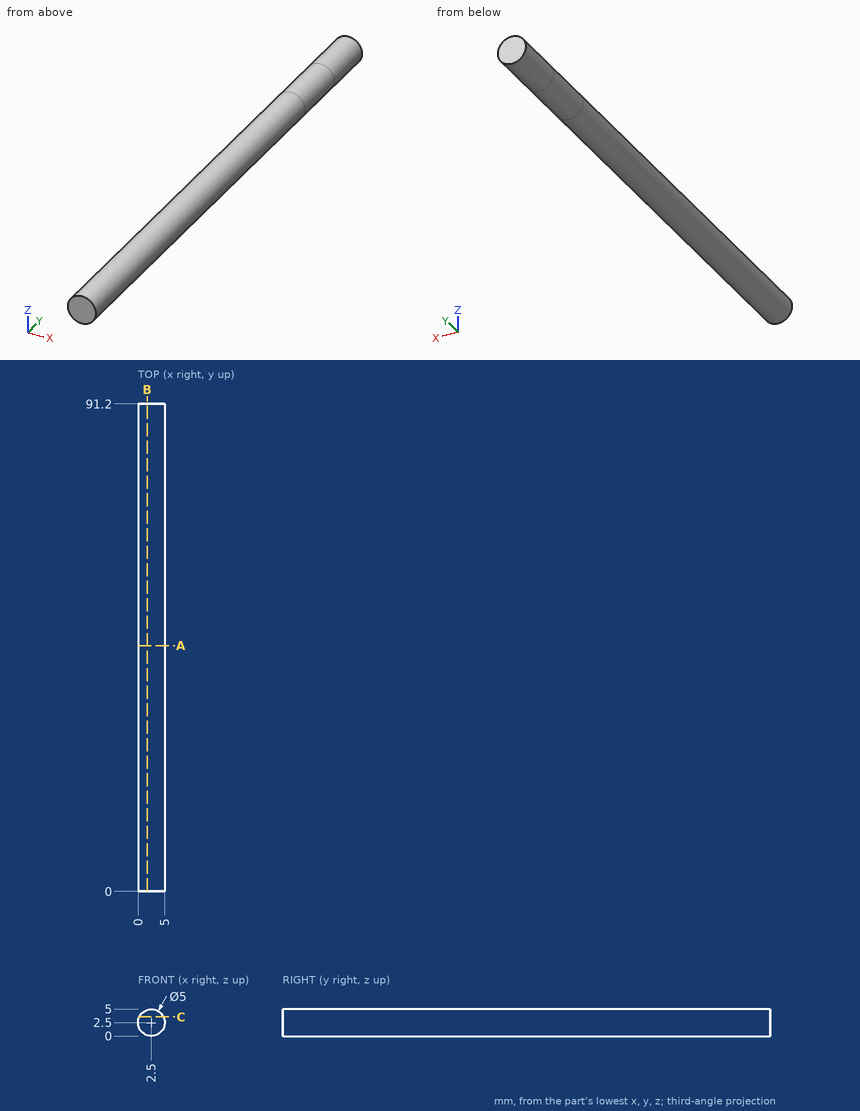
The drawing under review shows one solid part. Ordinate dimensions are in mm from its lowest x, y, z. Round coordinates to 2 decimals unless told otherwise and drop trailing zeros. Order: outer loops, then holes, each group sorted by start corner. A loop starts at its lowest first (then second) coordinate and runs counter-clockwise, first axis right, second up. Notation, with made-up numbers: (37, 58.25) -> (47, 58.25) arc R27 ccw to (47, 84.25) -> close; hole circle Ø8 at (-38.5, 50). An arc over 180 degrees is marked (long way). Use a Markdown table: item, result.
Item 1: For line 1 along X through (y, z) = (68, 2.2); line 2 along Z through (x, y) = (2.1, 78); line 3 along X through (y, z) = (17, 4.3), list the stretches that pass through material, from the lowest coordinate up. Write a range as [from, to].
Resolved:
| item | result |
|---|---|
| line 1 | x = [0.02, 4.98] |
| line 2 | z = [0.03, 4.97] |
| line 3 | x = [0.77, 4.23] |
Item 2: Take a section at A-A (y = 46). State the section outline as (x, z) points, plus the area to 3 significant figures.
Resolved:
| item | result |
|---|---|
| outline | circle Ø5 at (2.5, 2.5) |
| area | 19.6 mm² |
Item 3: Take a section at C-C (z = 3.6). State the section outline as (x, y) points (3 decimals).
Resolved:
| item | result |
|---|---|
| outline | (0.255, 0) -> (4.745, 0) -> (4.745, 91.2) -> (0.255, 91.2) -> close |
Item 4: Take a section at B-B (x = 1.7). State the section outline as (y, z) points.
Resolved:
| item | result |
|---|---|
| outline | (0, 0.13) -> (91.2, 0.13) -> (91.2, 4.87) -> (0, 4.87) -> close |
